Model file for the job. Use its own axes, mm. A direction names the side the tool comes from. Give positions to 0.01 mm unless a question says otherwise; leave off trailing zeros. Order: outer loops, then holes, each group sorted by start corner. A loop starts at its lowest first (then second) coordinate and runs counter-clockwise, first axis right, second up. Notation, with made-up numbers: (-25, 7) - (18, 7) arc R14 cw to (18, 11) - close; hole circle Ø10 at (29.25, 32.5). An arc over 180 degrees is marked (long way). Return JSON: item names as keys, results as strings. Group by question number.
from build123d import *

# Parameters (mm, degrees)
SKETCH1_R               = 3.9
SKETCH1_R_2             = 2.55
BOSS_EXTRUDE1_DEPTH     = 0.65
SKETCH3_W               = 3.9
SKETCH3_H               = 6
CUT_EXTRUDE1_DEPTH      = 4.9
CUT_EXTRUDE1_DEPTH_BACK = 4.9
SKETCH4_W               = 3
SKETCH4_H               = 9
CUT_EXTRUDE2_DEPTH      = 4.9
CUT_EXTRUDE2_DEPTH_BACK = 4.9
SKETCH6_R               = 2.55
CUT_EXTRUDE3_DEPTH      = 5.5
SKETCH7_W               = 4
SKETCH7_H               = 8
CUT_EXTRUDE5_DEPTH      = 4.9
CUT_EXTRUDE5_DEPTH_BACK = 4.9
SKETCH9_R               = 2.25
CUT_EXTRUDE6_DEPTH      = 5.5
CUT_EXTRUDE6_TAPER      = -20


with BuildPart() as part:
    # Sketch1 → Boss-Extrude1 (new body)
    with BuildSketch(Plane(origin=(0, 0, 0), x_dir=(1, 0, 0), z_dir=(0, 1, 0))):
        Circle(SKETCH1_R)
        Circle(SKETCH1_R_2, mode=Mode.SUBTRACT)
    extrude(amount=BOSS_EXTRUDE1_DEPTH)

    # Sketch2 → Revolve1 (revolve)
    with BuildSketch(Plane.XY):
        Polygon((-2.55, 0), (-3.05, 0), (-3.45, -0.3), (-3.05, -0.6), (-3.45, -0.9), (-3.05, -1.2), (-3.45, -1.5), (-3.05, -3.75), (-2.55, -3.75), align=None)
    revolve(axis=Axis((0, 0, 0), (0, -1, 0)))

    # Sketch3 → Cut-Extrude1 (cut, two sides)
    with BuildSketch(Plane.XY) as cut_extrude1_sk:
        with Locations((0, -3)):
            Rectangle(SKETCH3_W, SKETCH3_H)
    extrude(amount=CUT_EXTRUDE1_DEPTH, mode=Mode.SUBTRACT)
    extrude(cut_extrude1_sk.sketch, amount=-CUT_EXTRUDE1_DEPTH_BACK, mode=Mode.SUBTRACT)

    # Sketch4 → Cut-Extrude2 (cut, two sides)
    with BuildSketch(Plane(origin=(0, 0, 0), x_dir=(0, 0, -1), z_dir=(1, 0, 0))) as cut_extrude2_sk:
        with Locations((-3.15, -4.5)):
            Rectangle(SKETCH4_W, SKETCH4_H)
        with Locations((3.15, -4.5)):
            Rectangle(SKETCH4_W, SKETCH4_H)
    extrude(amount=CUT_EXTRUDE2_DEPTH, mode=Mode.SUBTRACT)
    extrude(cut_extrude2_sk.sketch, amount=-CUT_EXTRUDE2_DEPTH_BACK, mode=Mode.SUBTRACT)


with BuildPart() as body_2:
    # Sketch5 → Revolve2 (revolve)
    with BuildSketch(Plane(origin=(0, 0, 0), x_dir=(0, 0, -1), z_dir=(1, 0, 0))):
        Polygon((3.1, -4.95), (2.7, -4.7025), (3.1, -4.455), (2.7, -4.2075), (3.1, -3.96), (2.7, -3.7125), (3.1, -3.465), (2.7, -3.2175), (3.1, -2.97), (2.7, -2.7225), (3.1, -2.475), (2.7, -2.2275), (3.1, -1.98), (2.7, -1.7325), (3.1, -1.485), (2.7, -1.2375), (3.1, -0.99), (2.7, -0.7425), (3.1, -0.495), (2.7, -0.2475), (3.1, 0), (0, 0), (0, -6.45), (2.791521213, -6.45), align=None)
    revolve(axis=Axis((0, 0, 0), (0, -1, 0)))

    # Sketch6 → Cut-Extrude3 (cut)
    with BuildSketch(Plane(origin=(0, 0, 0), x_dir=(1, 0, 0), z_dir=(0, 1, 0))):
        Circle(SKETCH6_R)
    extrude(amount=-CUT_EXTRUDE3_DEPTH, mode=Mode.SUBTRACT)

    # Sketch7 → Cut-Extrude5 (cut, two sides)
    with BuildSketch(Plane.XY) as cut_extrude5_sk:
        with Locations((3.65, -4)):
            Rectangle(SKETCH7_W, SKETCH7_H)
        with Locations((-3.65, -4)):
            Rectangle(SKETCH7_W, SKETCH7_H)
    extrude(amount=CUT_EXTRUDE5_DEPTH, mode=Mode.SUBTRACT)
    extrude(cut_extrude5_sk.sketch, amount=-CUT_EXTRUDE5_DEPTH_BACK, mode=Mode.SUBTRACT)

    # Sketch9 → Cut-Extrude6 (cut)
    with BuildSketch(Plane(origin=(0, -5.5, 0), x_dir=(1, 0, 0), z_dir=(0, 1, 0))):
        Circle(SKETCH9_R)
    extrude(amount=-CUT_EXTRUDE6_DEPTH, taper=CUT_EXTRUDE6_TAPER, mode=Mode.SUBTRACT)


with BuildPart() as part_1:
    add(part.part)

    # Combine1: union body 2
    add(body_2.part)


solid = part_1.part
(1) Pull direction Y, two halves, no side cores. Call faces 3 (the face through (0.03, -0.34, 2.85)), 4 (the face through (0.026, -5.689, 2.948)), 5 (the face through (2.4, -1.9, 1.65)): released by +Y, released by -Y, zero draft, split by the parting line, or undercut.
(2) Drop flat-ended pins along their axis: pin 1 Ø3 at (y, z) = (-4.5, -3) entering from +X; pin 2 Ø1 at (x, y) = (3, -1) entering from +Z; pin 3 Ø1.5 at (y, z) = (-3.5, 1.5) entering from +X; pin 4 Ø4 at (x, z) = (0, 1) entering from -Y. Give the stop position or say it passes through.
(3) Slice it at A-A (z = 3.25). Give the cut face in (x, y).
(4) Drill centre lines: L1, parallel to Y at x = -2, z = -1.75; L2, parallel to X at y = -3, z = 1.5; L3, parallel to X at y = -0.5, z = -0.5. Where is each one in solid material? Low to high.
(5) 3-axis set-ups, long thin cutter, end or side, ignore diameter. For faces 1 (the face through (-2.4, -1.9, -1.65)), 2 (the face through (-2.7, -3.75, 0)): which of +Z, -Z, +X, -X, +Y, -Y reach the whole face in a straight line?
Result set:
{
 "1": {"face 3": "undercut", "face 4": "released by -Y", "face 5": "zero draft"},
 "2": {"pin 1": "stops at x = 1.65", "pin 2": "stops at z = 1.65", "pin 3": "stops at x = 3.04", "pin 4": "stops at y = -6.45"},
 "3": {"outline": "(-2.16, 0) - (2.16, 0) - (2.16, 0.65) - (-2.16, 0.65) - close"},
 "4": {"L1": "y = 0 to 0.65", "L2": "x = -2.81 to -2.06, 2.06 to 2.81", "L3": "x = -3.14 to -2.5, 2.5 to 3.14"},
 "5": {"face 1": "-Z, +X, -X, -Y", "face 2": "+Z, -Z, +X, -X, -Y"}
}
